from build123d import *

# Parameters (mm, degrees)
SKETCH1_W                    = 30
SKETCH1_H                    = 30
BOSS_EXTRUDE1_DEPTH          = 30
F_3_0_3_DIAMETER_HOLE1_D     = 3
F_3_0_3_DIAMETER_HOLE1_DEPTH = 2.5
F_3_0_3_DIAMETER_HOLE1_TIP   = 0.901290929
F_3_0_3_DIAMETER_HOLE2_D     = 3
F_3_0_3_DIAMETER_HOLE2_DEPTH = 2.5
F_3_0_3_DIAMETER_HOLE2_TIP   = 0.901290929
F_3_0_3_DIAMETER_HOLE3_D     = 3
F_3_0_3_DIAMETER_HOLE3_DEPTH = 2.5
F_3_0_3_DIAMETER_HOLE3_TIP   = 0.901290929
F_3_0_3_DIAMETER_HOLE4_D     = 3
F_3_0_3_DIAMETER_HOLE4_DEPTH = 2.5
F_3_0_3_DIAMETER_HOLE4_TIP   = 0.901290929
F_3_0_3_DIAMETER_HOLE5_D     = 3
F_3_0_3_DIAMETER_HOLE5_DEPTH = 2.5
F_3_0_3_DIAMETER_HOLE5_TIP   = 0.901290929
F_3_0_3_DIAMETER_HOLE6_D     = 3
F_3_0_3_DIAMETER_HOLE6_DEPTH = 2.5
F_3_0_3_DIAMETER_HOLE6_TIP   = 0.901290929
SKETCH14_W                   = 17.836209409
SKETCH14_H                   = 14.772604036
CUT_EXTRUDE1_DEPTH           = 5.320508076
FILLET1_R                    = 2.5


with BuildPart() as part:
    # Sketch1 → Boss-Extrude1 (new body)
    with BuildSketch(Plane(origin=(0, 0, 0), x_dir=(1, 0, 0), z_dir=(0, 1, 0))):
        with Locations((15, 15)):
            Rectangle(SKETCH1_W, SKETCH1_H)
    extrude(amount=BOSS_EXTRUDE1_DEPTH)

    # Ø3.0 (3) Diameter Hole1
    with Locations(Plane(origin=(7.5, 22.5, 0), x_dir=(1, 0, 0), z_dir=(0, 0, 1))):
        with Locations((0, 0), (7.5, 0), (15, 0), (15, -15), (7.5, -15), (0, -15)):
            Hole(F_3_0_3_DIAMETER_HOLE1_D / 2, depth=F_3_0_3_DIAMETER_HOLE1_DEPTH)
            with Locations((0, 0, -(F_3_0_3_DIAMETER_HOLE1_DEPTH + F_3_0_3_DIAMETER_HOLE1_TIP / 2))):  # 118° drill point
                Cone(0, F_3_0_3_DIAMETER_HOLE1_D / 2, F_3_0_3_DIAMETER_HOLE1_TIP, mode=Mode.SUBTRACT)

    # Ø3.0 (3) Diameter Hole2
    with Locations(Plane(origin=(7.5, 30, -22.5), x_dir=(0, 0, 1), z_dir=(0, 1, 0))):
        with Locations((0, 0), (7.5, 7.5), (0, 15), (15, 15), (15, 0)):
            Hole(F_3_0_3_DIAMETER_HOLE2_D / 2, depth=F_3_0_3_DIAMETER_HOLE2_DEPTH)
            with Locations((0, 0, -(F_3_0_3_DIAMETER_HOLE2_DEPTH + F_3_0_3_DIAMETER_HOLE2_TIP / 2))):  # 118° drill point
                Cone(0, F_3_0_3_DIAMETER_HOLE2_D / 2, F_3_0_3_DIAMETER_HOLE2_TIP, mode=Mode.SUBTRACT)

    # Ø3.0 (3) Diameter Hole3
    with Locations(Plane(origin=(15, 15, -30), x_dir=(-1, 0, 0), z_dir=(0, 0, -1))):
        with Locations((0, 0)):
            Hole(F_3_0_3_DIAMETER_HOLE3_D / 2, depth=F_3_0_3_DIAMETER_HOLE3_DEPTH)
            with Locations((0, 0, -(F_3_0_3_DIAMETER_HOLE3_DEPTH + F_3_0_3_DIAMETER_HOLE3_TIP / 2))):  # 118° drill point
                Cone(0, F_3_0_3_DIAMETER_HOLE3_D / 2, F_3_0_3_DIAMETER_HOLE3_TIP, mode=Mode.SUBTRACT)

    # Ø3.0 (3) Diameter Hole4
    with Locations(Plane(origin=(7.5, 0, -7.5), x_dir=(0, 0, -1), z_dir=(0, -1, 0))):
        with Locations((0, 0), (15, 15)):
            Hole(F_3_0_3_DIAMETER_HOLE4_D / 2, depth=F_3_0_3_DIAMETER_HOLE4_DEPTH)
            with Locations((0, 0, -(F_3_0_3_DIAMETER_HOLE4_DEPTH + F_3_0_3_DIAMETER_HOLE4_TIP / 2))):  # 118° drill point
                Cone(0, F_3_0_3_DIAMETER_HOLE4_D / 2, F_3_0_3_DIAMETER_HOLE4_TIP, mode=Mode.SUBTRACT)

    # Ø3.0 (3) Diameter Hole5
    with Locations(Plane(origin=(30, 7.5, -7.5), x_dir=(0, 0, 1), z_dir=(1, 0, 0))):
        with Locations((0, 0), (-15, 0), (-15, -15), (0, -15)):
            Hole(F_3_0_3_DIAMETER_HOLE5_D / 2, depth=F_3_0_3_DIAMETER_HOLE5_DEPTH)
            with Locations((0, 0, -(F_3_0_3_DIAMETER_HOLE5_DEPTH + F_3_0_3_DIAMETER_HOLE5_TIP / 2))):  # 118° drill point
                Cone(0, F_3_0_3_DIAMETER_HOLE5_D / 2, F_3_0_3_DIAMETER_HOLE5_TIP, mode=Mode.SUBTRACT)

    # Ø3.0 (3) Diameter Hole6
    with Locations(Plane(origin=(0, 22.5, -7.5), x_dir=(0, 0, -1), z_dir=(-1, 0, 0))):
        with Locations((0, 0), (7.5, 7.5), (15, 15)):
            Hole(F_3_0_3_DIAMETER_HOLE6_D / 2, depth=F_3_0_3_DIAMETER_HOLE6_DEPTH)
            with Locations((0, 0, -(F_3_0_3_DIAMETER_HOLE6_DEPTH + F_3_0_3_DIAMETER_HOLE6_TIP / 2))):  # 118° drill point
                Cone(0, F_3_0_3_DIAMETER_HOLE6_D / 2, F_3_0_3_DIAMETER_HOLE6_TIP, mode=Mode.SUBTRACT)

    # Sketch14 → Cut-Extrude1 (cut, through all)
    with BuildSketch(Plane(origin=(17.505553499, -17.505553499, -17.505553499), x_dir=(0.816496581, 0.40824829, 0.40824829), z_dir=(-0.577350269, 0.577350269, 0.577350269))):
        with Locations((11.862983406, 20.967424405)):
            Rectangle(SKETCH14_W, SKETCH14_H)
    extrude(amount=-CUT_EXTRUDE1_DEPTH, mode=Mode.SUBTRACT)

    # Fillet1
    fillet1_edges = [part.edges().sort_by_distance(p)[0] for p in [
        (30, 30, -15),
        (11.258330249, 0, -30),
        (15, 30, -30),
        (0, 30, -15),
        (30, 0, -11.258330249),
        (15, 0, 0),
        (0, 0, -15),
        (15, 30, 0),
        (0, 15, -30),
        (30, 18.741669751, -30),
        (30, 15, 0),
        (0, 15, 0),
    ]]
    fillet(fillet1_edges, radius=FILLET1_R)


solid = part.part
Part model, mm, in its own coordinate system. A direction names the side the tool comes from. Coordinates: 2 decimals unless noted, no trailing zeros. Use a Markdown table: item, result. Add a question column.
Q1. Probe L1, parallel to X at y = 29.35, z = -7.5; L2, parallel to X at y = 23.5, z = -1.25; L3, parallel to Z at x = 7.5, y = 28.3. List the from-to ranges inside material, lowest first.
Q2. Which spindle directions (+Z, -Z, +X, -X, +Y, -Y) get a long thin tool onto all of the face, cutting with end or side? Do faces 4 (the cylindrical face through (1.3, 8.4, -23.7)), 5 (the cylindrical face through (15.175, 29.287, -29.248)), 6 (the cylindrical face through (23.51, 1.27, -23.61)), 7 (the cylindrical face through (16.2, 6.6, -1.3)), 8 (the cylindrical face through (23.987, 28.732, -7.305)). Say none if no direction does.
Q3. Mould opens along Z. For faces 1 (the cylindrical face through (28.7, 8.4, -6.3)), 2 (the flat face through (0, 12, -15)), 3 (the cylindrical face through (13.916, 0.713, -29.248)) say: +Z half, -Z half, draft (parallel to the pull), parting line (faces both ways), or undercut.
Q4. Pin check, flat tips, straight feed: P1, Ø2.5, axis at y = 7.5, z = -22.5, coming from the +X side; P2, Ø2.5, axis at x = 7.5, z = -22.5, coming from the +Y side; P3, Ø1.8, axis at x = 7.5, y = 22.5, coming from the +Z side. Stop position of each tip, or through.
Worked out:
| question | item | result |
|---|---|---|
| 1 | L1 | x = 0.82 to 6, 9 to 21, 24 to 29.18 |
| 1 | L2 | x = 0.33 to 6.38, 8.62 to 13.88, 16.12 to 21.38, 23.62 to 29.67 |
| 1 | L3 | z = -29.87 to -24, -21 to -9, -6 to -0.13 |
| 2 | face 4 | -X |
| 2 | face 5 | -Z, +X, -X, +Y |
| 2 | face 6 | -Y |
| 2 | face 7 | +Z |
| 2 | face 8 | +Y |
| 3 | face 1 | undercut |
| 3 | face 2 | draft |
| 3 | face 3 | -Z half |
| 4 | P1 | stops at x = 27.35 |
| 4 | P2 | stops at y = 27.35 |
| 4 | P3 | stops at z = -2.86 |
